```python
from build123d import *

# Parameters (mm, degrees)
RESSALTO_EXTRUS_O1_DEPTH      = 8
RESSALTO_EXTRUS_O2_DEPTH      = 12.3
CORTE_EXTRUS_O1_DEPTH         = 29.979993098687927
RESSALTO_EXTRUS_O3_DEPTH      = 9.3
RESSALTO_EXTRUS_O3_DEPTH_BACK = 12.3
CORTE_EXTRUS_O2_DEPTH         = 145.04110524430172
CORTE_EXTRUS_O5_START         = 3.75
ESBO_O10_W                    = 11
ESBO_O10_H                    = 3.4999999999999987
CORTE_EXTRUS_O5_DEPTH         = 149.21637788030614


with BuildPart() as part:
    # Esboço1 → Ressalto-extrusão1 (new body)
    with BuildSketch(Plane.XY):
        Polygon((-8, 10.499999999999998), (8, 10.499999999999998), (8.000000000000004, -10.500000000000002), (-8, -10.500000000000002), align=None)
    extrude(amount=RESSALTO_EXTRUS_O1_DEPTH)

    # Esboço2 → Ressalto-extrusão2 (add)
    with BuildSketch(Plane(origin=(0, 10.499999999999998, 0), x_dir=(1, 0, 0), z_dir=(0, 1, 0))):
        Polygon((-6.000000000000002, -1.750000000000001), (5.999999999999998, -1.750000000000001), (5.999999999999998, -6.25), (-6, -6.25), align=None)
    extrude(amount=RESSALTO_EXTRUS_O2_DEPTH)

    # Esboço3 → Corte-extrusão1 (cut, through all)
    with BuildSketch(Plane(origin=(8.000000000000002, 1.32e-15, 0), x_dir=(0, 0, -1), z_dir=(1, 1.7e-16, 0))):
        with BuildLine():
            Line((12.302112688752674, -8.041249801298202), (15.759799941349684, -18.709266127928004))
            Line((15.759799941349684, -18.709266127928004), (-12.82894273367674, -20.250050884769166))
            Line((-12.82894273367674, -20.250050884769166), (-17.748760130002903, -20.25005088476917))
            Line((-17.748760130002903, -20.25005088476917), (-21.504856301930886, -7.075521773543869))
            Line((-21.504856301930886, -7.075521773543869), (-8, -7.499999999999983))
            ThreePointArc((-8, -7.499999999999983), (-7.121320343559643, -9.621320343559647), (-4.999999999999979, -10.500000000000004))
            Line((-4.999999999999979, -10.500000000000004), (-3.0000000000000213, -10.500000000000004))
            ThreePointArc((-3.0000000000000213, -10.500000000000004), (-0.8786796564403576, -9.621320343559647), (0, -7.499999999999983))
            Line((0, -7.499999999999983), (12.302112688752674, -8.041249801298202))
        make_face()
    extrude(amount=-CORTE_EXTRUS_O1_DEPTH, mode=Mode.SUBTRACT)

    # Esboço4 → Ressalto-extrusão3 (add, two sides: drawn at the far end of the back side and taken through both)
    with BuildSketch(Plane.XZ.offset(10.500000000000002).offset(-RESSALTO_EXTRUS_O3_DEPTH_BACK)):
        Polygon((-4.6499999999999995, 6.700000000000003), (4.650000000000001, 6.700000000000004), (4.650000000000001, 1.3000000000000025), (-4.649999999999998, 1.3000000000000025), align=None)
    extrude(amount=RESSALTO_EXTRUS_O3_DEPTH + RESSALTO_EXTRUS_O3_DEPTH_BACK)

    # Esboço8 → Revolução1 (revolve)
    with BuildSketch(Plane(origin=(0, 0, 0), x_dir=(0, 0, -1), z_dir=(1, 0, 0)), mode=Mode.PRIVATE) as revolu_o1_sk:
        with BuildLine():
            Line((0.6999999999999975, -15.150000000000004), (-1.3000000000000025, -15.150000000000002))
            Line((-1.3000000000000025, -15.150000000000002), (-6.700000000000003, -15.150000000000004))
            Line((-6.700000000000003, -15.150000000000004), (-125.70000000000003, -15.150000000000018))
            Line((-125.70000000000003, -15.150000000000018), (-125.7, -18.150000000000013))
            ThreePointArc((-125.7, -18.150000000000006), (-119.7371767478927, -18.359131245703352), (-113.80365649100945, -18.985497252888337))
            ThreePointArc((-113.80365649100945, -18.985497252888337), (-108.01923466009754, -19.596123836980453), (-102.20624616421328, -19.80000000000001))
            Line((-102.20624616421328, -19.800000000000015), (-6.700000000000003, -19.800000000000004))
            Line((-6.700000000000003, -19.800000000000004), (0.6999999999999981, -19.800000000000004))
            Line((0.6999999999999981, -19.800000000000004), (0.6999999999999975, -15.150000000000004))
        make_face()
        with BuildLine():
            Line((-125.7, -18.150000000000013), (-125.70000000000003, -15.150000000000018))
            Line((-125.70000000000003, -15.150000000000018), (-148.7, -15.15000000000002))
            ThreePointArc((-148.7, -15.15000000000002), (-147.82132034355962, -17.271320343559655), (-145.7, -18.15000000000001))
            Line((-145.7, -18.150000000000013), (-125.7, -18.150000000000013))
        make_face()
    revolve(revolu_o1_sk.sketch.rotate(Axis((0, -15.150000000000004, 6.700000000000003), (0, -1.1e-16, 1)), 180), axis=Axis((0, -15.150000000000004, 6.700000000000003), (0, -1.1e-16, 1)))

    # Esboço9 → Corte-extrusão2 (cut, through all)
    with BuildSketch(Plane.XY.offset(6.700000000000003)):
        with BuildLine():
            ThreePointArc((4.650000000000001, -15.150000000000004), (3.2880465325174466, -18.43804653251745), (6.2e-16, -19.800000000000004))
            Line((6.2e-16, -19.800000000000004), (4.650000000000002, -19.800000000000004))
            Line((4.650000000000002, -19.800000000000004), (4.650000000000002, -15.150000000000004))
        make_face()
        with BuildLine():
            Line((-4.649999999999999, -19.800000000000004), (8.9e-16, -19.800000000000004))
            ThreePointArc((4.1e-16, -19.800000000000004), (-3.2880465325174453, -18.43804653251745), (-4.649999999999998, -15.150000000000004))
            Line((-4.649999999999999, -15.150000000000004), (-4.649999999999999, -19.800000000000004))
        make_face()
    extrude(amount=-CORTE_EXTRUS_O2_DEPTH, mode=Mode.SUBTRACT)

    # Esboço10 → Corte-extrusão5 (cut, through all)
    with BuildSketch(Plane(origin=(0, 10.499999999999998, 0), x_dir=(1, 0, 0), z_dir=(0, 1, 0)).offset(CORTE_EXTRUS_O5_START)):
        with Locations((-1.78e-15, -4.000000000000001)):
            Rectangle(ESBO_O10_W, ESBO_O10_H)
    extrude(amount=CORTE_EXTRUS_O5_DEPTH, mode=Mode.SUBTRACT)


solid = part.part
```
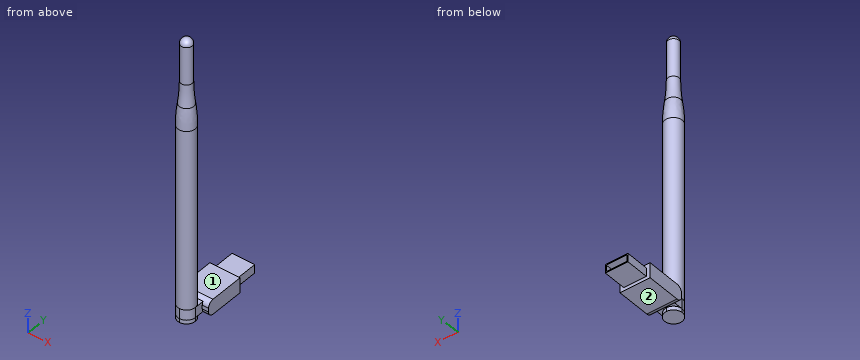
Design review of the part built by this model. Coordinates are the model's own, in mm. Face numbers are marked on the shaded views. A direction names the side the tool comes from. Coordinates: 2 decimals unless noted, no trailing zeros. Order: outer loops, then holes, each group sorted by start corner. A loop starts at its lowest first (then second) coordinate and runs counter-clockwise, first axis right, second up.
1) Wall thickness on line 1 along Z through (x, y) = (-4, 19.5); line 2 along Y through (x, z) = (0.5, 18); line 3 along Z through (x, y) = (3.75, -10): over which ranges is each line inside the solid? List them lowest first.
2) For the marked faces 1 and 2, list the 3-axis set-ups (+Z, -Z, +X, -X, +Y, -Y) from which the entire face can be reached by the end or side of a thin tool; tool diameter is ignored.
3) Clearance check with flat-ended pins moving along their axes: pin 1 (2 mm diameter, centred on x = 6.5, z = 4.5, fed in from -Y); pin 2 (1 mm diameter, centred on x = 2, y = 14.5, fed in from +Z); pin 3 (5 mm diameter, centred on y = -14, z = 114.5, fed in from +X). State where each tip first meets the part, or that it passes through.
4) Take a section at C-C, the plane z = 116.5. Give the boundary of the cut face in (x, y), and give its area (3 significant figures).
5) Take a section at A-A, the plane z = 42.5. Give the boundary of the cut face in (x, y), and give its area (3 significant figures).
6) Take a section at B-B, the plane y = -6. Give the boundary of the cut face in (x, z), and give its area (3 significant figures).
Returned:
1. line 1: z = 1.75 to 2.25, 5.75 to 6.25
1. line 2: y = -19.77 to -10.53
1. line 3: z = 1.3 to 6.7
2. face 1: +Z, +X, -X, +Y
2. face 2: -Z, +X, -X, +Y
3. pin 1: stops at y = -10.5
3. pin 2: stops at z = 6.25
3. pin 3: stops at x = 4.04
4. outline: circle Ø7 at (0, -15.15)
4. area: 38.5 mm2
5. outline: circle Ø9.3 at (0, -15.15)
5. area: 67.9 mm2
6. outline: (-8, 0) - (8, 0) - (8, 8) - (-8, 8) - close
6. area: 128 mm2
